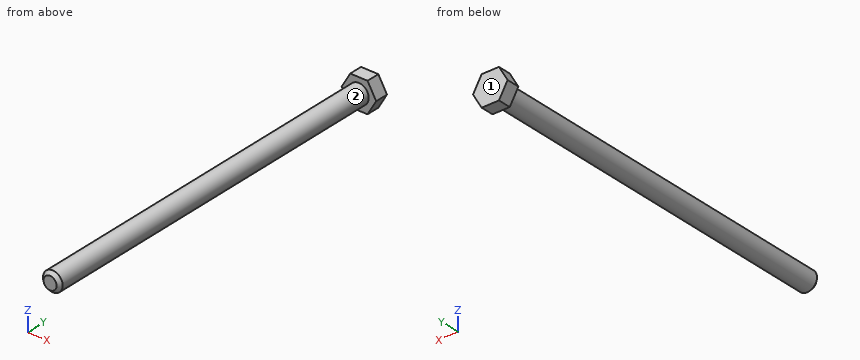
```python
from build123d import *

# Parameters (mm, degrees)
EXTRUDE1_DEPTH = 6.223
SKETCH2_R      = 4.699
EXTRUDE2_DEPTH = 177.8
CHAMFER1_SIZE  = 1.5875


with BuildPart() as part:
    # Sketch1 → Extrude1 (new body)
    with BuildSketch(Plane(origin=(0, 0, 0), x_dir=(1, 0, 0), z_dir=(0, 1, 0))):
        Polygon((8.263556668, 0), (4.131778334, 7.15645), (-4.131778334, 7.15645), (-8.263556668, 0), (-4.131778334, -7.15645), (4.131778334, -7.15645), align=None)
    extrude(amount=-EXTRUDE1_DEPTH)

    # Sketch2 → Extrude2 (add)
    with BuildSketch(Plane.XZ.offset(6.223)):
        Circle(SKETCH2_R)
    extrude(amount=EXTRUDE2_DEPTH)

    # Chamfer1
    chamfer1_edges = [part.edges().sort_by_distance(p)[0] for p in [
        (-4.699, -184.023, 0),
    ]]
    chamfer(chamfer1_edges, length=CHAMFER1_SIZE)


solid = part.part
```
CAD build for the part. Positions are in the model's coordinates, mm. Face numbers are marked on the shaded views. A direction names the side the tool comes from. Coordinates: 2 decimals unless noted, no trailing zeros. Order: outer loops, then holes, each group sorted by start corner. A loop starts at its lowest first (then second) coordinate and runs counter-clockwise, first axis right, second up. Notation, with made-up numbers: (-3, -30) -> (55, -30) arc R32 cw to (55, 3) -> close; hole circle Ø6 at (10.25, 19.5). An arc over 180 degrees is marked (long way). Use one line per item in the form item = value. Start each with the question number.
1) Drop flat-ended pins along their axis: pin 1 (1.5 mm diameter, centred on x = 5, z = -2, fed in from +Y); pin 2 (8 mm diameter, centred on x = -3, y = -45, fed in from -Z); pin 3 (8 mm diameter, centred on y = -32, z = -1.5, fed in from -X); pin 4 (4 mm diameter, centred on y = -139, z = -3, fed in from +X). Give the stop position or say it passes through.
2) Band-saw the part on A-A on x = 0. Give the cut face in (y, z), then the cut area to 3 significant figures.
3) Band-saw the part on B-B on y = -41. Give the cut face in (x, z), then the cut area to 3 significant figures.
4) Tool access for the marked faces 1 and 2: list every direction of +Z, -Z, +X, -X, +Y, -Y with a clear straight run to the whole face (end or side of a thin tool).
5) Drill centre lines: L1, parallel to Y at x = 2.5, z = -5.75; L2, parallel to Z at x = 0.5, y = -33.5; L3, parallel to X at y = -54, z = 3.5. Where is each one in solid material? Low to high. Write a range as [from, to].
Entries:
q1.pin_1 = 0
q1.pin_2 = -4.7
q1.pin_3 = -4.7
q1.pin_4 = 4.59
q2.outline = (-184.02, -3.11) -> (-182.44, -4.7) -> (-6.22, -4.7) -> (-6.22, -7.16) -> (0, -7.16) -> (0, 7.16) -> (-6.22, 7.16) -> (-6.22, 4.7) -> (-182.44, 4.7) -> (-184.02, 3.11) -> close
q2.area = 1,760 mm2
q3.outline = circle Ø9.4 at (0, 0)
q3.area = 69.4 mm2
q4.face_1 = +Z, -Z, +X, -X, +Y
q4.face_2 = -Y
q5.L1 = [-6.22, 0]
q5.L2 = [-4.67, 4.67]
q5.L3 = [-3.14, 3.14]
